from build123d import *

# Parameters (mm, degrees)
F3_R      = 20.0994613734
F4_DEPTH  = 5.08
F5_DEPTH  = 7.62
F6_R      = 5.08
F8_D      = 4.6999906
F8_DEPTH  = 2.54
F8_TIP    = 1.4120196307
F9_R      = 10.0000054
F10_DEPTH = 81.281


with BuildPart() as f2:
    # F0 (on Right) → F2 (revolve)
    with BuildSketch(Plane.YZ):
        with BuildLine():
            Line((-10.16, 0), (0, 0))
            Line((0, 0), (0, 68.58))
            Line((0, 68.58), (-38.1, 68.58))
            ThreePointArc((-38.1, 68.58), (-21.0473280724, 36.4062482775), (-20.32, 0))
            Line((-20.32, 0), (-10.16, 0))
        make_face()
    revolve(axis=Axis((0, 0, 21.4434694499), (0, 0, 1)))

    # F3 (on Top) → F4 (join)
    with BuildSketch(Plane.XY):
        Circle(F3_R)
    extrude(amount=-F4_DEPTH)

    # F5 (add): a face of the model
    f5_faces = [f2.faces().sort_by_distance(p)[0] for p in [
        (0, 0, 68.58),
    ]]
    extrude(f5_faces, amount=F5_DEPTH)

    # F6
    f6_edges = [f2.edges().sort_by_distance(p)[0] for p in [
        (0, 38.1, 76.2),
        (0, 38.1, 68.58),
    ]]
    fillet(f6_edges, radius=F6_R)

    # F8
    with Locations(Plane.XY.offset(76.2)):
        with Locations((14.499971, 0.168066554), (-14.499971, 0.168066554), (0, -14.5009449819)):
            Hole(F8_D / 2, depth=F8_DEPTH)
            with Locations((0, 0, -(F8_DEPTH + F8_TIP / 2))):  # 118° drill point
                Cone(0, F8_D / 2, F8_TIP, mode=Mode.SUBTRACT)

    # F9 (on face) → F10 (cut, through all)
    with BuildSketch(Plane.XY.offset(76.2)):
        Circle(F9_R)
    extrude(amount=-F10_DEPTH, mode=Mode.SUBTRACT)


solid = f2.part
Check sheet for the modelled part. Datum: model origin and axes. Units: mm. A direction names the side the tool comes from. Round coordinates to 2 decimals unless told otherwise and drop trailing zeros. Loops run counter-clockwise (first coordinate to the right, second up) from the corner with the lowest first, then second, coordinate; pieces in that order, holes last. Notation, with made-up numbers: (62.5, 42.25) - (97.5, 42.25) arc R23 cw to (97.5, 72.25) - close; hole circle Ø8 at (-21.5, 53.25). An arc over 180 degrees is marked (long way). Answer as CSV lines item,"result". Start each with the question number.
Item 1: Section check A-A (z = 37.5). Record the boundary of the cut face in (x, y).
Item 2: Set-up check for faces 1 (the cylindrical face through (-16.741, 0.874, 74.912)), 2 (the flat face through (8, 7, 76.2)), 3 (the cylindrical face through (-15.95, -12.23, -2.5)): record each of +Z, -Z, +X, -X, +Y, -Y from which the full face is reachable in a straight line by a thin tool's end or side.
Item 3: Depth check by flat-ended pin: P1, Ø3, axis at x = -11.5, z = 35.5, coming from the -Y side; P2, Ø4, axis at x = 0, y = -14.5, coming from the +Z side; P3, Ø1.5, axis at y = 10, z = 61, coming from the +X side. Enter the tip coordinate at first touch or a pass-through.
Item 4: Scan lines: line 1 (Y direction, x = 0, z = 58); line 2 (Y direction, x = 8.5, z = -1); line 3 (X direction, y = 6, z = 14). Record each from-to range of solid material in increasing order. Write a range as [from, to].
Report:
1,outline,"circle Ø42.68 at (0, 0); hole circle Ø20 at (0, 0)"
2,face 1,"+Z"
2,face 2,"+Z, +X, -X, +Y, -Y"
2,face 3,"-Z"
3,P1,"stops at y = -18.36"
3,P2,"stops at z = 73.45"
3,P3,"stops at x = 31.22"
4,line 1,"y = [-30.27, -10], [10, 30.27]"
4,line 2,"y = [-18.21, -5.27], [5.27, 18.21]"
4,line 3,"x = [-17.58, -8], [8, 17.58]"
